Check sheet for the modelled part. Datum: model origin and axes. Units: mm. Coordinates: 2 decimals unless noted, no trailing zeros. Order: outer loops, then holes, each group sorted by start corner. A loop starts at its lowest first (then second) coordinate and runs counter-clockwise, first axis right, second up.
1. Cross-section at D-D (z = 1.5). Enter the section's corners in (x, y).
2. Cross-section at C-C (x = 0). Enter the section's corners in (y, z).
3. Cross-section at A-A (y = 30). Enter the section's corners in (x, z).
4. Thickness scan on line 1 (Y direction, x = 30, z = 0.85); line 2 (Y direction, x = 0, z = 1.85); line 3 (X direction, y = 31.5, z = 1.15). Record the ranges inside material, lowest first.
5. Cross-section at B-B (y = -12.8). Enter the section's corners in (x, z), then the cut area to 3 significant figures.
```python
from build123d import *

# Parameters (mm, degrees)
F0_W     = 120
F0_H     = 120
F1_DEPTH = 3
F2_R     = 5.5
F3_DEPTH = 3.001
F5_D     = 6


with BuildPart() as f1:
    # F0 (on Top) → F1 (new body)
    with BuildSketch(Plane.XY):
        Rectangle(F0_W, F0_H)
    extrude(amount=F1_DEPTH)

    # F2 (on face) → F3 (cut, through all)
    with BuildSketch(Plane.XY.offset(3)):
        with Locations((0, 12.8)):
            Circle(F2_R)
        with Locations((0, -12.8)):
            Circle(F2_R)
    extrude(amount=-F3_DEPTH, mode=Mode.SUBTRACT)

    # F5 (through all)
    with Locations(Plane.XY.offset(3)):
        with Locations((-30, -30), (-30, 30), (30, 30), (30, -30)):
            Hole(F5_D / 2)


solid = f1.part
```
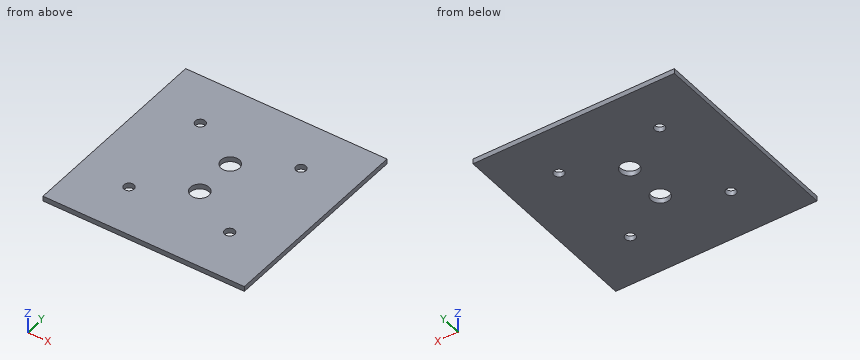
Data:
1. outline: (-60, -60) - (60, -60) - (60, 60) - (-60, 60) - close; hole circle Ø6 at (-30, -30); hole circle Ø6 at (-30, 30); hole circle Ø11 at (0, -12.8); hole circle Ø11 at (0, 12.8); hole circle Ø6 at (30, -30); hole circle Ø6 at (30, 30)
2. outline: (-60, 0) - (-18.3, 0) - (-18.3, 3) - (-60, 3) - close; (-7.3, 0) - (7.3, 0) - (7.3, 3) - (-7.3, 3) - close; (18.3, 0) - (60, 0) - (60, 3) - (18.3, 3) - close
3. outline: (-60, 0) - (-33, 0) - (-33, 3) - (-60, 3) - close; (-27, 0) - (27, 0) - (27, 3) - (-27, 3) - close; (33, 0) - (60, 0) - (60, 3) - (33, 3) - close
4. line 1: y = -60 to -33, -27 to 27, 33 to 60
4. line 2: y = -60 to -18.3, -7.3 to 7.3, 18.3 to 60
4. line 3: x = -60 to -32.6, -27.4 to 27.4, 32.6 to 60
5. outline: (-60, 0) - (-5.5, 0) - (-5.5, 3) - (-60, 3) - close; (5.5, 0) - (60, 0) - (60, 3) - (5.5, 3) - close
5. area: 327 mm2
